Autodesk Inventor part; units mm, degrees
ref_plane "YZ Plane" through (0, 0, 0) normal (1, 0, 0) x (0, 1, 0)
ref_plane "XZ Plane" through (0, 0, 0) normal (0, 1, 0) x (-1, 0, 0)
ref_plane "XY Plane" through (0, 0, 0) normal (0, 0, 1) x (1, 0, 0)
sketch "Esboço1" plane through (0, 0, 0) normal (0, 0, 1) x (1, 0, 0)
  line L0 (0, 0) -> (160, 0)
  line L1 (160, 0) -> (160, 32.5)
  line L2 (0, 32.5) -> (0, 0)
  line L3 (20, 165) -> (140, 165)
  line L4 (160, 145) -> (160, 130)
  line L5 (0, 130) -> (0, 145)
  arc A0 (20, 165) -> (0, 145) centre (20, 145) ccw
  arc A1 (160, 145) -> (140, 165) centre (140, 145) ccw
  line L6 (127.5, 130) -> (127.5, 45)
  line L7 (32.5, 45) -> (32.5, 130)
  line L8 (12.5, 45) -> (32.5, 45)
  line L9 (127.5, 45) -> (147.5, 45)
  line L10 (160, 130) -> (127.5, 130)
  line L11 (32.5, 130) -> (0, 130)
  arc A2 (12.5, 45) -> (0, 32.5) centre (12.5, 32.5) ccw
  arc A3 (160, 32.5) -> (147.5, 45) centre (147.5, 32.5) ccw
  line L12 (20, 148) -> (20, 145)
  line L13 (20, 145) -> (140, 145)
  line L14 (140, 145) -> (140, 148)
  line L15 (140, 148) -> (20, 148)
  point P0 (0, 165)
  point P1 (160, 165)
  dimension "d3" = 160
  dimension "d4" = 165
  dimension "d6" = 20
  dimension "d12" = 95
  dimension "d14" = 85
  dimension "d15" = 35
  dimension "d16" = 12.5
  dimension "d17" = 12.5
  dimension "d73" = 3
  dimension "d74" = 32.5
extrude "Extrusão1" add sketch "Esboço1" along normal blind 2.5
sketch "Esboço2" plane through (0, 0, 0) normal (0, 0, -1) x (-1, 0, 0)
  line L0 (-10.5, 30.486) -> (-10.5, 10)
  line L1 (-10.5, 10) -> (0, 10)
  line L2 (0, 10) -> (0, 30.486)
  line L3 (0, 30.486) -> (-10.5, 30.486)
  line L4 (0, 32.5) -> (0, 0)
  line L5 (0, 0) -> (-160, 0)
  line L6 (-160, 30.486) -> (-160, 10)
  line L7 (-160, 10) -> (-149.5, 10)
  line L8 (-149.5, 10) -> (-149.5, 30.486)
  line L9 (-149.5, 30.486) -> (-160, 30.486)
  line L10 (-160, 0) -> (-160, 32.5)
  circle A0 centre (-5.25, 10) radius 2
  circle A1 centre (-154.75, 30.486) radius 2
  circle A2 centre (-154.75, 10) radius 2
  circle A3 centre (-5.25, 30.486) radius 2
  line L11 (-98.69, 46.742) -> (-98.69, 10)
  line L12 (-98.69, 10) -> (-61.31, 10)
  line L13 (-61.31, 10) -> (-61.31, 46.742)
  line L14 (-61.31, 46.742) -> (-98.69, 46.742)
  circle A4 centre (-98.69, 46.742) radius 1.75
  circle A5 centre (-61.31, 46.742) radius 1.75
  circle A6 centre (-98.69, 10) radius 1.75
  circle A7 centre (-61.31, 10) radius 1.75
  line L15 (-100.26, 112.382) -> (-115.5, 112.382)
  line L16 (-115.5, 112.382) -> (-115.5, 71.742)
  line L17 (-115.5, 71.742) -> (-100.26, 71.742)
  line L18 (-100.26, 71.742) -> (-100.26, 112.382)
  line L19 (-127.5, 45) -> (-127.5, 130)
  circle A8 centre (-100.26, 112.382) radius 0.75
  circle A9 centre (-115.5, 112.382) radius 0.75
  circle A10 centre (-115.5, 71.742) radius 0.75
  circle A11 centre (-100.26, 71.742) radius 0.75
  line L20 (-68.8516, 140.982) -> (-85.9516, 140.982)
  line L21 (-85.9516, 140.982) -> (-85.9516, 123.882)
  line L22 (-85.9516, 123.882) -> (-68.8516, 123.882)
  line L23 (-68.8516, 123.882) -> (-68.8516, 140.982)
  circle A12 centre (-83.0586, 138.0895) radius 1.25
  circle A13 centre (-71.7446, 126.775) radius 1.25
  line L24 (-32.5, 130) -> (-32.5, 45)
  line L25 (-83.5, 75.089) -> (-38.5, 75.089)
  line L26 (-38.5, 75.089) -> (-38.5, 109.089)
  line L27 (-38.5, 109.089) -> (-83.5, 109.089)
  line L28 (-83.5, 109.089) -> (-83.5, 75.089)
  line L29 (-38.5, 98.658) -> (-35.5, 98.658)
  line L30 (-35.5, 98.658) -> (-35.5, 85.52)
  line L31 (-35.5, 85.52) -> (-38.5, 85.52)
  line L32 (-83.5, 98.658) -> (-86.5, 98.658)
  line L33 (-86.5, 98.658) -> (-86.5, 85.52)
  line L34 (-86.5, 85.52) -> (-83.5, 85.52)
  line L35 (-68.8516, 133.932) -> (-75.9016, 133.932)
  line L36 (-78.9016, 133.932) -> (-85.9516, 133.932)
  line L37 (-85.9516, 130.932) -> (-78.9016, 130.932)
  line L38 (-75.9016, 130.932) -> (-68.8516, 130.932)
  line L39 (-75.9016, 140.982) -> (-75.9016, 133.932)
  line L40 (-75.9016, 130.932) -> (-75.9016, 123.882)
  line L41 (-78.9016, 123.882) -> (-78.9016, 130.932)
  line L42 (-78.9016, 133.932) -> (-78.9016, 140.982)
  dimension "d20" = 20.486
  dimension "d21" = 10.5
  dimension "d22" = 10
  dimension "d23" = 20.486
  dimension "d24" = 10.5
  dimension "d26" = 4
  dimension "d27" = 4
  dimension "d28" = 4
  dimension "d29" = 4
  dimension "d30" = 36.742
  dimension "d35" = 3.5
  dimension "d36" = 3.5
  dimension "d37" = 3.5
  dimension "d38" = 3.5
  dimension "d39" = 15.24
  dimension "d40" = 40.64
  dimension "d42" = 12
  dimension "d43" = 1.5
  dimension "d44" = 1.5
  dimension "d45" = 1.5
  dimension "d46" = 1.5
  dimension "d47" = 17.1
  dimension "d48" = 17.1
  dimension "d50" = 2.5
  dimension "d51" = 2.5
  dimension "d52" = 2.893
  dimension "d53" = 2.8925
  dimension "d54" = 2.893
  dimension "d55" = 2.893
  dimension "d56" = 36.3516
  dimension "d57" = 41.5484
  dimension "d58" = 11.5
  dimension "d59" = 45
  dimension "d60" = 34
  dimension "d64" = 6
  dimension "d65" = 3
  dimension "d66" = 10.431
  dimension "d67" = 10.431
  dimension "d68" = 3
  dimension "d79" = 3
  dimension "d80" = 3
  dimension "d81" = 7.05
  dimension "d82" = 7.05
  dimension "d83" = 28.347
  dimension "d84" = 25
  dimension "d85" = 10
  dimension "d86" = 50.81
  dimension "d87" = 50.81
  dimension "d88" = 37.38
extrude "Extrusão2" cut sketch "Esboço2" against normal through all contours A3 L3 | L3 A3 | A0 L1 | L1 A0 | A2 L7 | L7 A2 | A1 L9 | L9 A1 | L14 A4 L11 | L11 A4 L14 | A6 L12 L11 | L11 L12 A6 | A5 L13 L14 | L14 L13 A5 | A7 L13 L12 | L12 L13 A7 | A9 L16 L15 | L15 L16 A9 | A8 L18 L15 | L15 L18 A8 | A10 L17 L16 | L16 L17 A10 | A11 L17 L18 | L18 L17 A11 | L39 L35 L23 L38 L40 L22 L41 L37 L21 L36 L42 L20 | A12 | A13 | L34 L33 L32 L28 | L26 L29 L30 L31
The listing builds one solid part. Answer for the finished solid, in the listing's coordinates (mm). A direction names the side the tool comes from. Coordinates: 2 decimals unless noted, no trailing zeros. Order: outer loops, then holes, each group sorted by start corner. A loop starts at its lowest first (then second) coordinate and runs counter-clockwise, first axis right, second up. Notation, with made-up numbers: M 60,37 L 64,37 A13 cw 64,42 Z; hole C 58,55 d1. An arc over 180 degrees is marked long. Answer as a JSON object with one key per item and string values. Group by question number.
1. Straight lines are drawn through the part: line 1 (X direction, y = 92.5, z = 0.7); line 2 (Y direction, x = 115.5, z = 1.45); line 3 (Y direction, x = 21.5, z = 1.6). For each, find the intervals that lie inside material, in ascending order.
2. A tool of negligible diameter and unlimited length cuts with its end or side. For faces 5 (the cylindrical face through (156.241, 41.435, 1.232)), 6 (the cylindrical face through (3.565, 41.241, 1.232)), 7 (the flat face through (79, 84, 0)), from which of +Z, -Z, +X, -X, +Y, -Y can it reach the whole face along a straight path? Write none if from no direction.
3. Section D-D on z = 2 is taken. State how many separate pieces and enclosed holes the cut face has, then the cut area to 3 significant figures.
4. Section A-A on x = 22 is taken. Write down the section's boundary in (y, z).
5. Section B-B on x = 54.5 is taken. Write down the section's boundary in (y, z).
6. A flat-ended cylindrical pin translates along its axis: P1, Ø4, axis at x = 99, y = 102, coming from the -Z side. Find the tip coordinate at first contact, or state that the pin passes through.
7. Determine the mould class of faces 1 (the cylindrical face through (5.51, 32.47, 1.23)), 2 (the cylindrical face through (5.703, 158.986, 1.232)), 3 (the flat face through (79, 84, 2.5)), 4 (the cylindrical face through (59.641, 10.526, 1.232)) for opening direction X: released by +X, released by -X, zero draft, split by the parting line, or undercut.
8. Section C-C on x = 5.25 is taken. Write down the section's boundary in (y, z).
Values follow:
{
 "1": {"line 1": "32.5 to 35.5, 38.5 to 83.5, 86.5 to 127.5", "line 2": "0 to 70.99, 72.49 to 111.63, 113.13 to 145, 148 to 165", "line 3": "0 to 45, 130 to 145, 148 to 165"},
 "2": {"face 5": "+Z, -Z, +X", "face 6": "+Z, -Z, -X", "face 7": "-Z, +X, -X, +Y, -Y"},
 "3": {"separate pieces": "1", "enclosed holes": "18", "area": "20,000 mm2"},
 "4": {"outline": "M 0,0 L 45,0 L 45,2.5 L 0,2.5 Z; M 130,0 L 145,0 L 145,2.5 L 130,2.5 Z; M 148,0 L 165,0 L 165,2.5 L 148,2.5 Z"},
 "5": {"outline": "M 0,0 L 145,0 L 145,2.5 L 0,2.5 Z; M 148,0 L 165,0 L 165,2.5 L 148,2.5 Z"},
 "6": {"P1": "z = 0"},
 "7": {"face 1": "undercut", "face 2": "released by -X", "face 3": "zero draft", "face 4": "undercut"},
 "8": {"outline": "M 0,0 L 8,0 L 8,2.5 L 0,2.5 Z; M 12,0 L 28.49,0 L 28.49,2.5 L 12,2.5 Z; M 32.49,0 L 42.68,0 L 42.68,2.5 L 32.49,2.5 Z; M 130,0 L 158.51,0 L 158.51,2.5 L 130,2.5 Z"}
}
